```python
from build123d import *

# Parameters (mm, degrees)
F1_DEPTH  = 6.35
F2_R      = 11.0236
F3_DEPTH  = 25.4
F4_R      = 11.0236
F5_DEPTH  = 25.4
F7_DEPTH  = 6.35
F9_DEPTH  = 6.35
F11_DEPTH = 25.4


with BuildPart() as f1:
    # F0 (on Top) → F1 (new body)
    with BuildSketch(Plane.XY):
        with BuildLine():
            ThreePointArc((39.9699173868, 45.3715771437), (21.4086371945, 56.0642096985), (0, 56.787927047))
            ThreePointArc((0, 56.787927047), (10.5518009423, 52.4172279893), (14.9225, 41.865427047))
            ThreePointArc((14.9225, 41.865427047), (14.5429525108, 38.5212472494), (13.4236173036, 35.3471830552))
            ThreePointArc((13.4236173036, 35.3471830552), (25.7159889241, 42.956648129), (39.9699173868, 45.3715771437))
        make_face()
        with BuildLine():
            Line((11.4783198204, -9.5356793335), (13.9973004553, -5.1726768904))
            ThreePointArc((13.9973004553, -5.1726768904), (14.6893791954, -2.6273836992), (14.9225, 0))
            ThreePointArc((14.9225, 0), (11.4076836995, 9.6200706267), (2.518980635, 14.7083562239))
            Line((2.518980635, 14.7083562239), (-2.518980635, 14.7083562239))
            ThreePointArc((-2.518980635, 14.7083562239), (-12.923264088, 7.46125), (-13.9973004553, -5.1726768904))
            Line((-13.9973004553, -5.1726768904), (-11.4783198204, -9.5356793335))
            ThreePointArc((-11.4783198204, -9.5356793335), (0, -14.9225), (11.4783198204, -9.5356793335))
        make_face()
        with BuildLine():
            ThreePointArc((-59.2778971096, 11.9291752723), (-59.2573484392, -9.4916811784), (-49.179787451, -28.3939635235))
            ThreePointArc((-49.179787451, -28.3939635235), (-49.4383993618, -13.9384908074), (-37.3233671298, -6.048397932))
            ThreePointArc((-37.3233671298, -6.048397932), (-50.0595430032, 0.7923756272), (-59.2778971096, 11.9291752723))
        make_face()
        with BuildLine():
            Line((24.7782035426, -11.39703419), (13.9973004553, -5.1726768904))
            ThreePointArc((13.9973004553, -5.1726768904), (12.923264088, -7.46125), (11.4783198204, -9.5356793335))
            Line((11.4783198204, -9.5356793335), (11.4007932052, -9.6699593699))
            Line((11.4007932052, -9.6699593699), (22.205423221, -15.9080154181))
            ThreePointArc((22.205423221, -15.9080154181), (23.2940753375, -13.5397474451), (24.7782035426, -11.39703419))
        make_face()
        with BuildLine():
            ThreePointArc((-2.518980635, 14.7083562239), (0, 14.9225), (2.518980635, 14.7083562239))
            Line((2.518980635, 14.7083562239), (2.6740338653, 14.7083562239))
            Line((2.6740338653, 14.7083562239), (2.6740338653, 27.1844683202))
            ThreePointArc((2.6740338653, 27.1844683202), (0.0787275795, 26.9431347225), (-2.518980635, 27.1570708231))
            Line((-2.518980635, 27.1570708231), (-2.518980635, 14.7083562239))
        make_face()
        with BuildLine():
            Line((-22.2592229077, -15.7600366331), (-11.4783198204, -9.5356793335))
            ThreePointArc((-11.4783198204, -9.5356793335), (-12.923264088, -7.46125), (-13.9973004553, -5.1726768904))
            Line((-13.9973004553, -5.1726768904), (-14.0748270705, -5.038396854))
            Line((-14.0748270705, -5.038396854), (-24.8794570864, -11.2764529022))
            ThreePointArc((-24.8794570864, -11.2764529022), (-23.372802917, -13.4033872774), (-22.2592229077, -15.7600366331))
        make_face()
        with BuildLine():
            ThreePointArc((0, 56.787927047), (-14.8688676772, 43.1294603729), (-2.518980635, 27.1570708231))
            Line((-2.518980635, 27.1570708231), (-2.518980635, 27.4083562239))
            Line((-2.518980635, 27.4083562239), (2.6740338653, 27.4083562239))
            Line((2.6740338653, 27.4083562239), (2.6740338653, 27.1844683202))
            ThreePointArc((2.6740338653, 27.1844683202), (5.574874939, 28.0233977281), (8.2474275307, 29.429151665))
            ThreePointArc((8.2474275307, 29.429151665), (10.6805834625, 32.5236842879), (13.4236173036, 35.3471830552))
            ThreePointArc((13.4236173036, 35.3471830552), (14.5429525108, 38.5212472494), (14.9225, 41.865427047))
            ThreePointArc((14.9225, 41.865427047), (10.5518009423, 52.4172279893), (0, 56.787927047))
        make_face()
        with BuildLine():
            ThreePointArc((19.3079797228, -57.3007524159), (37.8487112447, -46.5725285201), (49.179787451, -28.3939635235))
            ThreePointArc((49.179787451, -28.3939635235), (36.7902868106, -35.845664366), (23.8997498262, -29.2987851232))
            ThreePointArc((23.8997498262, -29.2987851232), (24.3435540791, -43.7490237562), (19.3079797228, -57.3007524159))
        make_face()
        with BuildLine():
            ThreePointArc((-21.334023363, -20.9327135235), (-21.5671441676, -18.3053298244), (-22.2592229077, -15.7600366331))
            Line((-22.2592229077, -15.7600366331), (-22.4768424484, -15.8856793335))
            Line((-22.4768424484, -15.8856793335), (-25.0733496986, -11.388396854))
            Line((-25.0733496986, -11.388396854), (-24.8794570864, -11.2764529022))
            ThreePointArc((-24.8794570864, -11.2764529022), (-27.0564118024, -9.183715544), (-29.6101067191, -7.5720940751))
            ThreePointArc((-29.6101067191, -7.5720940751), (-33.5066285492, -7.0121855382), (-37.3233671298, -6.048397932))
            ThreePointArc((-37.3233671298, -6.048397932), (-49.4383993618, -13.9384908074), (-49.179787451, -28.3939635235))
            ThreePointArc((-49.179787451, -28.3939635235), (-32.3942961625, -35.3467416663), (-21.334023363, -20.9327135235))
        make_face()
        with BuildLine():
            ThreePointArc((51.179023363, -20.9327135235), (41.3258319318, -6.8976461249), (24.7782035426, -11.39703419))
            Line((24.7782035426, -11.39703419), (24.9958230834, -11.5226768904))
            Line((24.9958230834, -11.5226768904), (22.3993158332, -16.0199593699))
            Line((22.3993158332, -16.0199593699), (22.205423221, -15.9080154181))
            ThreePointArc((22.205423221, -15.9080154181), (21.4815368634, -18.8396821842), (21.3626791884, -21.8570575899))
            ThreePointArc((21.3626791884, -21.8570575899), (22.8260450868, -25.5114987497), (23.8997498262, -29.2987851232))
            ThreePointArc((23.8997498262, -29.2987851232), (36.7902868106, -35.845664366), (49.179787451, -28.3939635235))
            ThreePointArc((49.179787451, -28.3939635235), (50.6705515058, -24.794940724), (51.179023363, -20.9327135235))
        make_face()
        with BuildLine():
            ThreePointArc((13.4236173036, 35.3471830552), (10.6805834625, 32.5236842879), (8.2474275307, 29.429151665))
            ThreePointArc((8.2474275307, 29.429151665), (11.2322891672, 32.0411364205), (13.4236173036, 35.3471830552))
        make_face()
        with BuildLine():
            ThreePointArc((-37.3233671298, -6.048397932), (-33.5066285492, -7.0121855382), (-29.6101067191, -7.5720940751))
            ThreePointArc((-29.6101067191, -7.5720940751), (-33.3645826899, -6.2931204488), (-37.3233671298, -6.048397932))
        make_face()
        with BuildLine():
            ThreePointArc((23.8997498262, -29.2987851232), (22.8260450868, -25.5114987497), (21.3626791884, -21.8570575899))
            ThreePointArc((21.3626791884, -21.8570575899), (22.1322935227, -25.7480159717), (23.8997498262, -29.2987851232))
        make_face()
        with BuildLine():
            Line((24.9958230834, -11.5226768904), (24.7782035426, -11.39703419))
            ThreePointArc((24.7782035426, -11.39703419), (23.2940753375, -13.5397474451), (22.205423221, -15.9080154181))
            Line((22.205423221, -15.9080154181), (22.3993158332, -16.0199593699))
            Line((22.3993158332, -16.0199593699), (24.9958230834, -11.5226768904))
        make_face()
        with BuildLine():
            Line((-22.4768424484, -15.8856793335), (-22.2592229077, -15.7600366331))
            ThreePointArc((-22.2592229077, -15.7600366331), (-23.372802917, -13.4033872774), (-24.8794570864, -11.2764529022))
            Line((-24.8794570864, -11.2764529022), (-25.0733496986, -11.388396854))
            Line((-25.0733496986, -11.388396854), (-22.4768424484, -15.8856793335))
        make_face()
        with BuildLine():
            Line((-2.518980635, 14.7083562239), (2.518980635, 14.7083562239))
            ThreePointArc((2.518980635, 14.7083562239), (0, 14.9225), (-2.518980635, 14.7083562239))
        make_face()
        with BuildLine():
            ThreePointArc((-13.9973004553, -5.1726768904), (-12.923264088, -7.46125), (-11.4783198204, -9.5356793335))
            Line((-11.4783198204, -9.5356793335), (-13.9973004553, -5.1726768904))
        make_face()
        with BuildLine():
            Line((-2.518980635, 27.4083562239), (-2.518980635, 27.1570708231))
            ThreePointArc((-2.518980635, 27.1570708231), (0.0787275795, 26.9431347225), (2.6740338653, 27.1844683202))
            Line((2.6740338653, 27.1844683202), (2.6740338653, 27.4083562239))
            Line((2.6740338653, 27.4083562239), (-2.518980635, 27.4083562239))
        make_face()
        with BuildLine():
            ThreePointArc((11.4783198204, -9.5356793335), (12.923264088, -7.46125), (13.9973004553, -5.1726768904))
            Line((13.9973004553, -5.1726768904), (11.4783198204, -9.5356793335))
        make_face()
    extrude(amount=F1_DEPTH)

    # F2 (on face) → F3 (cut)
    with BuildSketch(Plane.XY.offset(6.35)):
        with Locations((0, 41.865427047)):
            Circle(F2_R)
        with Locations((36.256523363, -20.9327135235)):
            Circle(F2_R)
        with Locations((-36.256523363, -20.9327135235)):
            Circle(F2_R)
    extrude(amount=-F3_DEPTH, mode=Mode.SUBTRACT)

    # F4 (on face) → F5 (cut)
    with BuildSketch(Plane.XY.offset(6.35)):
        Circle(F4_R)
    extrude(amount=-F5_DEPTH, mode=Mode.SUBTRACT)

    # F6 (on Top) → F7 (join)
    with BuildSketch(Plane.XY):
        with BuildLine():
            Line((-2.518980635, 20.9327135235), (-2.518980635, 27.1570708231))
            ThreePointArc((-2.518980635, 27.1570708231), (-21.6236198706, 12.5506950245), (-24.8794570864, -11.2764529022))
            Line((-24.8794570864, -11.2764529022), (-19.4771420784, -8.1574248781))
            ThreePointArc((-19.4771420784, -8.1574248781), (-17.1752258506, 9.9886362226), (-2.518980635, 20.9327135235))
        make_face()
        with BuildLine():
            ThreePointArc((2.6740338653, 20.9464122721), (17.2380256432, 9.8798637911), (19.387751999, -8.2848555402))
            Line((19.387751999, -8.2848555402), (24.7782035426, -11.39703419))
            ThreePointArc((24.7782035426, -11.39703419), (21.6810306616, 12.4512566175), (2.6740338653, 27.1844683202))
            Line((2.6740338653, 27.1844683202), (2.6740338653, 20.9464122721))
        make_face()
        with BuildLine():
            ThreePointArc((16.8031082131, -12.788987394), (-0.0627997926, -19.8685000137), (-16.868771364, -12.6478579833))
            Line((-16.868771364, -12.6478579833), (-22.2592229077, -15.7600366331))
            ThreePointArc((-22.2592229077, -15.7600366331), (-0.057410791, -25.0019516419), (22.205423221, -15.9080154181))
            Line((22.205423221, -15.9080154181), (16.8031082131, -12.788987394))
        make_face()
    extrude(amount=F7_DEPTH)

    # F8 (on Top) → F9 (join)
    with BuildSketch(Plane.XY):
        with BuildLine():
            Line((-11.469233202, 6.8651486084), (-9.5382659064, 10.7402523643))
            ThreePointArc((-9.5382659064, 10.7402523643), (-11.469233202, 13.7334678675), (-14.9203554134, 14.6153574454))
            Line((-14.9203554134, 14.6153574454), (-18.1496096475, 10.3096855748))
            ThreePointArc((-18.1496096475, 10.3096855748), (-14.0887724556, 9.9850523749), (-11.469233202, 6.8651486084))
        make_face()
        with BuildLine():
            Line((11.6800096966, 6.5000730107), (14.0704643438, 2.8902544008))
            ThreePointArc((14.0704643438, 2.8902544008), (17.6281486563, 3.0659133811), (20.1174485398, 5.6137280988))
            Line((20.1174485398, 5.6137280988), (18.0032544366, 10.5631802361))
            ThreePointArc((18.0032544366, 10.5631802361), (15.6916952426, 7.2087086672), (11.6800096966, 6.5000730107))
        make_face()
        with BuildLine():
            Line((-0.2107764946, -13.3652216191), (-4.5321984374, -13.6305067652))
            ThreePointArc((-4.5321984374, -13.6305067652), (-6.1589154543, -16.7993812486), (-5.1970931264, -20.2290855441))
            Line((-5.1970931264, -20.2290855441), (0.146355211, -20.8728658109))
            ThreePointArc((0.146355211, -20.8728658109), (-1.602922787, -17.1937610422), (-0.2107764946, -13.3652216191))
        make_face()
    extrude(amount=F9_DEPTH)

    # F10 (on face) → F11 (cut)
    with BuildSketch(Plane.XY.offset(6.35)):
        Polygon((-45.3443394157, -5.8470536995), (-50.9034361544, -0.1712185392), (-58.0193315347, -3.7043041955), (-56.8581000013, -11.5637063766), (-49.0245240646, -12.8879983994), align=None)
        Polygon((27.7358667489, -36.3458230021), (25.5999976818, -43.9980595801), (32.217687304, -48.3940629219), (38.4435134847, -43.4587058238), (35.6735960501, -36.0124840487), align=None)
        Polygon((13.3509280145, 48.9004824481), (17.6084726668, 42.1928767016), (25.3034384727, 44.1692781193), (25.8016442307, 52.0983671174), (18.4145865166, 55.0224122004), align=None)
    extrude(amount=-F11_DEPTH, mode=Mode.SUBTRACT)


solid = f1.part
```
For this review, take the finished solid that the model builds, in its own axes (mm). Coordinates: 2 decimals unless noted, no trailing zeros. Order: outer loops, then holes, each group sorted by start corner. A loop starts at its lowest first (then second) coordinate and runs counter-clockwise, first axis right, second up. Notation, with made-up numbers: (-30, 70.25) - (-25, 70.25) arc R15 ccw to (-25, 79.25) - close; hole circle Ø2 at (44.25, -16.5). An arc over 180 degrees is marked (long way). Answer as a JSON object with one key per item and string values. Group by question number.
1. We need section B-B on y = -33.5. State the section outline as (x, z) points, then the cut area to 3 significant figures.
2. We need section C-C on z = 1. Give the number of separate pieces and of enclosed holes in the cut face, then the cut area to 3 significant figures.
3. Clearance check with flat-ended pins moving along their axes: P1, Ø17.5, axis at x = 0, y = 0, coming from the -Z side; P2, Ø3, axis at y = 17, z = 4.5, coming from the -X side; P3, Ø3, axis at x = 36, z = 2.5, coming from the -Y side; P4, Ø4, axis at x = 36, y = -41, coming from the +Z side. State where each tip first meets the part, or that it passes through.
4. For probe 1 along X at (y, z) = (10, 0.5); probe 2 along X at (y, z) = (-21.5, 1.5); probe 3 along Y at (x, z) = (35, 4.25), list the stretches that pass through material, from the lowest coordinate up.
5. The part is to be moulded in two halves that separate along Y. For faces 1 (the flat face through (-9, 9, 0)), 2 (the flat face through (-57.447, -7.579, 3.219)), 3 (the cylindrical face through (-59.33, -9.2, 3.13)), say which applies: pulls with the +Y half, pulls with the -Y half, needs draft (parallel to the pull), parting line crosses it, or undercut.
6. We need section A-A on x = 44. State the section outline as (y, z) points, then the cut area to 3 significant figures.
Final values:
{
 "1": {"outline": "(-44.3, 0) - (-28.21, 0) - (-28.21, 6.35) - (-44.3, 6.35) - close; (24.61, 0) - (47.17, 0) - (47.17, 6.35) - (24.61, 6.35) - close", "area": "245 mm²"},
 "2": {"separate pieces": "1", "enclosed holes": "13", "area": "2,870 mm²"},
 "3": {"P1": "through", "P2": "x = -19.68", "P3": "y = -49.5", "P4": "z = 6.35"},
 "4": {"probe 1": "-59.71 to -58.15, -22.96 to -17.17, -14.12 to -4.64, 4.64 to 11.08, 17.17 to 22.95", "probe 2": "-54.28 to -47.27, -25.25 to -21.34, -14.4 to 14.49, 21.34 to 25.25, 47.27 to 51.17", "probe 3": "-49.1 to -46.19, -36.04 to -31.88, -9.98 to -6.06, 45.17 to 49.51"},
 "5": {"face 1": "needs draft", "face 2": "undercut", "face 3": "parting line crosses it"},
 "6": {"outline": "(-39.16, 0) - (-28.78, 0) - (-28.78, 6.35) - (-39.16, 6.35) - close; (-13.09, 0) - (-8.18, 0) - (-8.18, 6.35) - (-13.09, 6.35) - close", "area": "97.1 mm²"}
}
